Design review of the part built by this model. Coordinates are the model's own, in mm. Face numbers are marked on the shaded views. A direction names the side the tool comes from. Give positions to 0.01 mm unless a question says otherwise; leave off trailing zeros. Loops run counter-clockwise (first coordinate to the right, second up) from the corner with the lowest first, then second, coordinate; pieces in that order, holes last. Notation, with made-up numbers: (76.25, 62.25) - (98.25, 62.25) arc R8 cw to (98.25, 71.25) - close; hole circle Ø3 at (-16, -7.5). An arc over 180 degrees is marked (long way). Write each question's results on one line, items separated by ' | '.
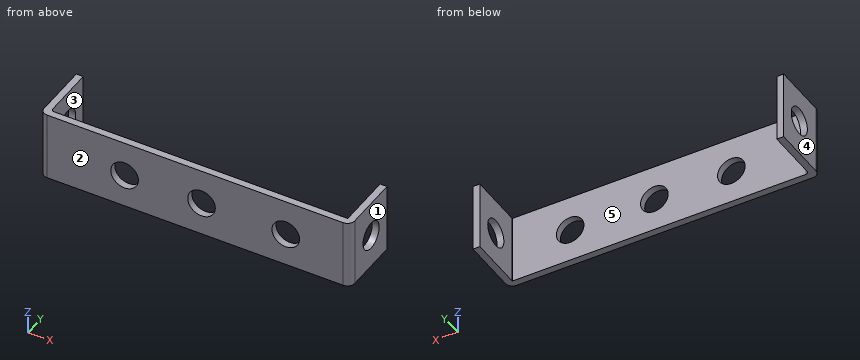
from build123d import *

# Parameters (mm, degrees)
CYLINDER030_R               = 2
CYLINDER030_DEPTH           = 10
CYLINDER030_PITCH_ANGLE     = 90
CYLINDER030_PLACEMENT_ANGLE = 7e-06
CYLINDER031_R               = 2
CYLINDER031_DEPTH           = 10
CYLINDER031_PITCH_ANGLE     = 90
CYLINDER031_PLACEMENT_ANGLE = 7e-06
CYLINDER026_R               = 2
CYLINDER026_DEPTH           = 2
CYLINDER026_ROLL_ANGLE      = -88.507054
CYLINDER026_PITCH_ANGLE     = -87.01751
CYLINDER026_PLACEMENT_ANGLE = -92.244015
CYLINDER028_R               = 2
CYLINDER028_DEPTH           = 2
CYLINDER028_PLACEMENT_ANGLE = 90.00001
CYLINDER029_R               = 2
CYLINDER029_DEPTH           = 2
CYLINDER029_ROLL_ANGLE      = 90
CYLINDER027_R               = 2
CYLINDER027_DEPTH           = 2
CYLINDER027_ROLL_ANGLE      = 90
CYLINDER025_R               = 2
CYLINDER025_DEPTH           = 2
CYLINDER025_ROLL_ANGLE      = -88.507054
CYLINDER025_PITCH_ANGLE     = -87.01751
CYLINDER025_PLACEMENT_ANGLE = -92.244015
PAD006_DEPTH                = 10


with BuildPart() as cylinder030:
    # Cylinder030 → Cylinder030 (new body)
    with BuildSketch(Plane.XY):
        Circle(CYLINDER030_R)
    extrude(amount=CYLINDER030_DEPTH)


with BuildPart() as cylinder030_1:
    # Cylinder030 pitch: moved
    add(cylinder030.part.rotate(Axis((0, 0, 0), (0, 1, 0)), CYLINDER030_PITCH_ANGLE))


with BuildPart() as cylinder030_2:
    # Cylinder030 placement: moved
    add(cylinder030_1.part.moved(Location((15.49, 3.9, 4.87))).rotate(Axis((15.49, 3.9, 4.87), (0, 0, 1)), CYLINDER030_PLACEMENT_ANGLE))


with BuildPart() as cylinder031:
    # Cylinder031 → Cylinder031 (new body)
    with BuildSketch(Plane.XY):
        Circle(CYLINDER031_R)
    extrude(amount=CYLINDER031_DEPTH)


with BuildPart() as cylinder031_1:
    # Cylinder031 pitch: moved
    add(cylinder031.part.rotate(Axis((0, 0, 0), (0, 1, 0)), CYLINDER031_PITCH_ANGLE))


with BuildPart() as cylinder031_2:
    # Cylinder031 placement: moved
    add(cylinder031_1.part.moved(Location((-28.4147, 3.9, 5.14))).rotate(Axis((-28.4147, 3.9, 5.14), (0, 0, 1)), CYLINDER031_PLACEMENT_ANGLE))


with BuildPart() as cylinder026:
    # Cylinder026 → Cylinder026 (new body)
    with BuildSketch(Plane.XY):
        Circle(CYLINDER026_R)
    extrude(amount=CYLINDER026_DEPTH)


with BuildPart() as cylinder026_1:
    # Cylinder026 roll: moved
    add(cylinder026.part.rotate(Axis((0, 0, 0), (1, 0, 0)), CYLINDER026_ROLL_ANGLE))


with BuildPart() as cylinder026_2:
    # Cylinder026 pitch: moved
    add(cylinder026_1.part.rotate(Axis((0, 0, 0), (0, 1, 0)), CYLINDER026_PITCH_ANGLE))


with BuildPart() as cylinder026_3:
    # Cylinder026 placement: moved
    add(cylinder026_2.part.moved(Location((-26, 5.29, 4.9))).rotate(Axis((-26, 5.29, 4.9), (0, 0, 1)), CYLINDER026_PLACEMENT_ANGLE))


with BuildPart() as cylinder028:
    # Cylinder028 → Cylinder028 (new body)
    with BuildSketch(Plane.XY):
        Circle(CYLINDER028_R)
    extrude(amount=CYLINDER028_DEPTH)


with BuildPart() as cylinder028_1:
    # Cylinder028 placement: moved
    add(cylinder028.part.moved(Location((-11.1555, 0, 4.86401))).rotate(Axis((-11.1555, 0, 4.86401), (1, 0, 0)), CYLINDER028_PLACEMENT_ANGLE))


with BuildPart() as cylinder029:
    # Cylinder029 → Cylinder029 (new body)
    with BuildSketch(Plane.XY):
        Circle(CYLINDER029_R)
    extrude(amount=CYLINDER029_DEPTH)


with BuildPart() as cylinder029_1:
    # Cylinder029 roll: moved
    add(cylinder029.part.rotate(Axis((0, 0, 0), (1, 0, 0)), CYLINDER029_ROLL_ANGLE))


with BuildPart() as cylinder029_2:
    # Cylinder029 placement: moved
    add(cylinder029_1.part.moved(Location((0, 0, 4.86401))))


with BuildPart() as cylinder027:
    # Cylinder027 → Cylinder027 (new body)
    with BuildSketch(Plane.XY):
        Circle(CYLINDER027_R)
    extrude(amount=CYLINDER027_DEPTH)


with BuildPart() as cylinder027_1:
    # Cylinder027 roll: moved
    add(cylinder027.part.rotate(Axis((0, 0, 0), (1, 0, 0)), CYLINDER027_ROLL_ANGLE))


with BuildPart() as cylinder027_2:
    # Cylinder027 placement: moved
    add(cylinder027_1.part.moved(Location((12.2129, 0, 4.81114))))


with BuildPart() as cylinder025:
    # Cylinder025 → Cylinder025 (new body)
    with BuildSketch(Plane.XY):
        Circle(CYLINDER025_R)
    extrude(amount=CYLINDER025_DEPTH)


with BuildPart() as cylinder025_1:
    # Cylinder025 roll: moved
    add(cylinder025.part.rotate(Axis((0, 0, 0), (1, 0, 0)), CYLINDER025_ROLL_ANGLE))


with BuildPart() as cylinder025_2:
    # Cylinder025 pitch: moved
    add(cylinder025_1.part.rotate(Axis((0, 0, 0), (0, 1, 0)), CYLINDER025_PITCH_ANGLE))


with BuildPart() as cylinder025_3:
    # Cylinder025 placement: moved
    add(cylinder025_2.part.moved(Location((25, 5.38, 4.9))).rotate(Axis((25, 5.38, 4.9), (0, 0, 1)), CYLINDER025_PLACEMENT_ANGLE))


with BuildPart() as cut019:
    # Sketch007 → Pad006 (new body)
    with BuildSketch(Plane.XY):
        with BuildLine():
            Line((20.546084, -1.208272), (-22.415471, -1.208272))
            ThreePointArc((-23.400725, -0.223018), (-23.112151, -0.919698), (-22.415471, -1.208272))
            Line((-23.400725, 7.776982), (-23.400725, -0.223018))
            Line((-23.400725, 7.776982), (-22.400725, 7.776982))
            Line((-22.400725, 7.776982), (-22.400725, 0.197829))
            ThreePointArc((-22.400725, 0.197829), (-22.286166, -0.07874), (-22.009596, -0.193299))
            Line((-22.009596, -0.193299), (20.555186, -0.193299))
            ThreePointArc((20.555186, -0.193299), (20.586324, -0.180401), (20.599222, -0.149263))
            Line((20.599222, 7.844865), (20.599222, -0.149263))
            Line((21.599222, 7.844865), (20.599222, 7.844865))
            Line((21.599222, 7.844865), (21.599222, -0.155135))
            ThreePointArc((20.546084, -1.208272), (21.290765, -0.899815), (21.599222, -0.155135))
        make_face()
    extrude(amount=PAD006_DEPTH)

    # Cut005: cut Cylinder025
    add(cylinder025_3.part, mode=Mode.SUBTRACT)

    # Cut006: cut Cylinder027
    add(cylinder027_2.part, mode=Mode.SUBTRACT)

    # Cut007: cut Cylinder029
    add(cylinder029_2.part, mode=Mode.SUBTRACT)

    # Cut008: cut Cylinder028
    add(cylinder028_1.part, mode=Mode.SUBTRACT)

    # Cut009: cut Cylinder026
    add(cylinder026_3.part, mode=Mode.SUBTRACT)

    # Cut018: cut Cylinder031
    add(cylinder031_2.part, mode=Mode.SUBTRACT)

    # Cut019: cut Cylinder030
    add(cylinder030_2.part, mode=Mode.SUBTRACT)


with BuildPart() as cut019_1:
    # Cut019 placement: moved
    add(cut019.part.moved(Location((-481.872341, 4.526565, -92.372143))))


solid = cut019_1.part
(1) Take a section at B-B on z = -90.5. Give the boundary of the cut face in (x, y), plus the area to 3 significant figures.
Answers below:
outline: (-505.27, 4.3) arc R0.99 ccw to (-504.29, 3.32) - (-461.33, 3.32) arc R1.05 ccw to (-460.27, 4.37) - (-460.27, 12.37) - (-461.27, 12.37) - (-461.27, 4.38) arc R0.04 cw to (-461.32, 4.33) - (-503.88, 4.33) arc R0.39 cw to (-504.27, 4.72) - (-504.27, 12.3) - (-505.27, 12.3) - close | area: 61.3 mm2
(2) Take a section at D-D on z = -88.75. Count the separate pieces of the cut face and the enclosed holes in it, plus the area to 3 significant figures.
Answers below:
separate pieces: 6 | enclosed holes: 0 | area: 45.9 mm2
(3) Take a section at C-C on y = 7.75. Give the boundary of the cut face in (x, z), plus the area to 3 significant figures.
Answers below:
outline: (-505.27, -92.37) - (-504.27, -92.37) - (-504.27, -89.11) - (-505.27, -89.11) - close; (-505.27, -85.35) - (-504.27, -85.35) - (-504.27, -82.37) - (-505.27, -82.37) - close; (-461.27, -92.37) - (-460.27, -92.37) - (-460.27, -89.38) - (-461.27, -89.38) - close; (-461.27, -85.62) - (-460.27, -85.62) - (-460.27, -82.37) - (-461.27, -82.37) - close | area: 12.5 mm2
(4) Take a section at A-A on y = 11. Give the boundary of the cut face in (x, z).
Answers below:
outline: (-505.27, -92.37) - (-504.27, -92.37) - (-504.27, -82.37) - (-505.27, -82.37) - close; (-461.27, -92.37) - (-460.27, -92.37) - (-460.27, -82.37) - (-461.27, -82.37) - close
(5) Draft analysis for pull direction X (two halves, no side actions). For the marked faces 1, 2 and 3, state which applies: pulls with the +X half, pulls with the -X half, needs draft (parallel to the pull), parting line crosses it, or undercut.
Answers below:
face 1: pulls with the +X half | face 2: needs draft | face 3: undercut
(6) Tool access review of the marked faces 4 and 5: name each direction out of +Z, -Z, +X, -X, +Y, -Y from which nothing blocks a thin tool from reaching the whole face with its end or side.
Answers below:
face 4: +Z, -Z, -X, +Y, -Y | face 5: +Z, -Z, +Y
(7) Wall thickness on line 1 along X through (y, z) = (9.5, -91); line 2 along Y through (x, z) = (-494.5, -84): over which ranges is each line inside the solid? List them lowest first. Write a range as from..to.
Answers below:
line 1: -505.27..-504.27, -461.27..-460.27 | line 2: 3.32..4.33
(8) Insertion check: P1, Ø1.5, axis at x = -474.5, z = -88, coming from the +Y side; P2, Ø5, axis at x = -469.5, y = 6, coming from the -Z side. Each pin has a flat end and moves straight along its axis. Give the tip position at first contact, or say it passes through.
Answers below:
P1: y = 4.33 | P2: z = -92.37
